Autodesk Inventor part; units mm, degrees
ref_plane "YZ Plane" through (0, 0, 0) normal (1, 0, 0) x (0, 1, 0)
ref_plane "XZ Plane" through (0, 0, 0) normal (0, 1, 0) x (-1, 0, 0)
ref_plane "XY Plane" through (0, 0, 0) normal (0, 0, 1) x (1, 0, 0)
sketch "Sketch2" plane through (0, 0, 0) normal (0, 0, 1) x (1, 0, 0)
  line L0 (0, 0) -> (99, 0)
  line L1 (99, 0) -> (99, 60)
  line L2 (99, 60) -> (0, 60)
  line L3 (0, 60) -> (0, 0)
  dimension "d2" = 99
  dimension "d3" = 60
extrude "Extrusion1" add sketch "Sketch2" along normal blind 60
sketch "Sketch3" plane through (0, 0, 0) normal (-1, 0, 0) x (0, 0, 1)
  circle A0 centre (30, 30) radius 4
  line L0 (0, 60) -> (60, 60)
  line L1 (0, 60) -> (0, 0)
  point P0 (30, 60)
  point P1 (0, 30)
  dimension "d6" = 8
extrude "Extrusion2" cut sketch "Sketch3" against normal through all
sketch "Sketch4" plane through (99, 0, 0) normal (1, 0, 0) x (0, 0, -1)
  line L0 (0, 60) -> (-60, 60)
  line L1 (-60, 60) -> (-50, 60)
  line L2 (-50, 60) -> (-50, 50)
  line L3 (-50, 50) -> (-60, 50)
  line L4 (-60, 50) -> (-60, 60)
  line L5 (0, 60) -> (-10, 60)
  line L6 (-10, 60) -> (-10, 50)
  line L7 (-10, 50) -> (0, 50)
  line L8 (0, 50) -> (0, 60)
  line L9 (0, 0) -> (-10, 0)
  line L10 (-10, 0) -> (-10, 10)
  line L11 (-10, 10) -> (0, 10)
  line L12 (0, 10) -> (0, 0)
  line L13 (-60, 0) -> (-50, 0)
  line L14 (-50, 0) -> (-50, 10)
  line L15 (-50, 10) -> (-60, 10)
  line L16 (-60, 10) -> (-60, 0)
  dimension "d9" = 10
  dimension "d10" = 10
  dimension "d11" = 10
  dimension "d12" = 10
  dimension "d13" = 10
  dimension "d14" = 10
  dimension "d15" = 10
  dimension "d16" = 10
extrude "Extrusion3" cut sketch "Sketch4" against normal blind 90
fillet "Fillet1" radius 3 8 edges at (54, 50, 60) (54, 60, 50) (54, 60, 10) (54, 50, 0) (54, 10, 60) (54, 0, 50) (54, 0, 10) (54, 10, 0)
fillet "Fillet2" radius 2 4 edges at (4.5, 60, 60) (4.5, 0, 60) (4.5, 60, 0) (4.5, 0, 0)
sketch "Sketch5" plane through (0, 2, 0) normal (-1, 0, 0) x (0, 0, 1)
  circle A0 centre (30, 28) radius 4
  circle A1 centre (30, 28) radius 17.5
  point P0 (0, -2)
  dimension "d21" = 35
extrude "Extrusion4" add sketch "Sketch5" along normal blind 3
sketch "Sketch6" plane through (0, 2, 0) normal (-1, 0, 0) x (0, 0, 1)
  line L0 (6.4, 4.4) -> (53.6, 4.4) construction
  line L1 (53.6, 4.4) -> (53.6, 51.6) construction
  line L2 (53.6, 51.6) -> (6.4, 51.6) construction
  line L3 (6.4, 51.6) -> (6.4, 4.4) construction
  circle A0 centre (6.4, 51.6) radius 2
  circle A1 centre (53.6, 51.6) radius 2
  circle A2 centre (53.6, 4.4) radius 2
  circle A3 centre (6.4, 4.4) radius 2
  circle A4 centre (30, 28) radius 4 construction
  point P0 (0, -2)
  point P1 (30, 51.6)
  point P2 (53.6, 28)
  dimension "d24" = 47.2
  dimension "d25" = 47.2
  dimension "d26" = 4
  dimension "d27" = 4
  dimension "d28" = 4
  dimension "d29" = 4
extrude "Extrusion5" cut sketch "Sketch6" against normal through all
properties material "Steel, Carbon"
Design review of the part built by this model. Coordinates are the model's own, in mm. A direction names the side the tool comes from. Give positions to 0.01 mm unless a question says otherwise; leave off trailing zeros. Loops run counter-clockwise (first coordinate to the right, second up) from the corner with the lowest first, then second, coordinate; pieces in that order, holes last. Notation, with made-up numbers: (-33.5, 17) - (17.5, 17) arc R27 ccw to (17.5, 46) - close; hole circle Ø6 at (1.25, 3). An arc over 180 degrees is marked (long way). Write item = value, one per line.
1) Take a section at B-B on y = 6.4. State the section outline as (x, z) points.
Result sheet:
outline = (0, 0) - (9, 0) - (9, 4.4) - (0, 4.4) - close; (0, 8.4) - (9, 8.4) - (9, 10) - (99, 10) - (99, 50) - (9, 50) - (9, 51.6) - (0, 51.6) - close; (0, 55.6) - (9, 55.6) - (9, 60) - (0, 60) - close
2) Take a section at C-C on x = 34. State the section outline as (y, z) points.
Result sheet:
outline = (0, 13) arc R3 ccw to (3, 10) - (10, 10) - (10, 3) arc R3 ccw to (13, 0) - (47, 0) arc R3 ccw to (50, 3) - (50, 10) - (57, 10) arc R3 ccw to (60, 13) - (60, 47) arc R3 ccw to (57, 50) - (50, 50) - (50, 57) arc R3 ccw to (47, 60) - (13, 60) arc R3 ccw to (10, 57) - (10, 50) - (3, 50) arc R3 ccw to (0, 47) - close; hole circle Ø8 at (30, 30)
3) To check wall thickness, follow line 1 (Y direction, x = 6.75, z = 6.4); line 2 (Y direction, x = 30, z = 30); line 3 (Z direction, x = 44.5, y = 55). State the ranges of each line that lie inside material, in increasing order.
Result sheet:
line_1 = 0 to 4.4, 8.4 to 51.6, 55.6 to 60
line_2 = 0 to 26, 34 to 60
line_3 = 10 to 50
4) Clearance check with flat-ended pins moving along their axes: pin 1 Ø6.5 at (y, z) = (6.4, 53.6) entering from -X; pin 2 Ø4 at (y, z) = (54, 54.5) entering from +X; pin 3 Ø5.5 at (x, z) = (40, 53.5) entering from -Y; pin 4 Ø3.5 at (y, z) = (53.6, 53.6) entering from -X. State where each tip first meets the part, or that it passes through.
Result sheet:
pin_1 = 0
pin_2 = 9
pin_3 = 10
pin_4 = through
5) Tool access review of faces 1 (the face through (53.37, 0.9, 10.86)), 2 (the face through (-1.479, 18.173, 17.102)), 3 (the face through (53.37, 49.14, 0.9)): name each direction out of +Z, -Z, +X, -X, +Y, -Y from which nothing blocks a thin tool from reaching the whole face with its end or side.
Result sheet:
face_1 = -Z, +X, -Y
face_2 = -X
face_3 = -Z, +X, +Y
6) Draft analysis for pull direction Y (two halves, no side actions). For faces 4 (the face through (4.437, 6.488, 51.602)), 5 (the face through (4.437, 51.648, 5.966)), 6 (the face through (55, 54, 50)), 7 (the face through (55, 10, 53)), state which applies: +Y half, -Y half, draft (parallel to the pull), parting line (faces both ways), or undercut.
Result sheet:
face_4 = undercut
face_5 = undercut
face_6 = draft
face_7 = -Y half
7) Take a section at A-A on z = 30. State the section outline as (x, y) points.
Result sheet:
outline = (-3, 12.5) - (0, 12.5) - (0, 0) - (99, 0) - (99, 26) - (-3, 26) - close; (-3, 34) - (99, 34) - (99, 60) - (0, 60) - (0, 47.5) - (-3, 47.5) - close
